The model under review builds one solid part; all positions refer to its coordinate system, in mm. A direction names the side the tool comes from. Give positions to 0.01 mm unless a question says otherwise; leave off trailing zeros. Loops run counter-clockwise (first coordinate to the right, second up) from the corner with the lowest first, then second, coordinate; pieces in that order, holes last. Notation, with made-up numbers: M 46,-34 L 75,-34 A21 cw 75,-10 Z; hole C 51,-30.75 d10. An arc over 180 degrees is marked long. Put each result on its own line as item: value. Start each with the question number.
from build123d import *

# Parameters (mm, degrees)
SKETCH1_W           = 10.541
SKETCH1_H           = 14.732
BOSS_EXTRUDE1_DEPTH = 1.524
SKETCH2_W           = 6.35
SKETCH2_H           = 9.652
BOSS_EXTRUDE2_DEPTH = 2.032
CUT_EXTRUDE1_DEPTH  = 6.35


with BuildPart() as part:
    # Sketch1 → Boss-Extrude1 (new body)
    with BuildSketch(Plane(origin=(0, 0, 0), x_dir=(0, 0, -1), z_dir=(1, 0, 0))):
        Rectangle(SKETCH1_W, SKETCH1_H)
    extrude(amount=BOSS_EXTRUDE1_DEPTH)

    # Sketch2 → Boss-Extrude2 (add)
    with BuildSketch(Plane(origin=(1.524, 0, 0), x_dir=(0, 0, -1), z_dir=(1, 0, 0))):
        Rectangle(SKETCH2_W, SKETCH2_H)
    extrude(amount=BOSS_EXTRUDE2_DEPTH)

    # Sketch3 → Cut-Extrude1 (cut)
    with BuildSketch(Plane.XY.offset(3.175)):
        Polygon((1.524, -4.826), (3.556, -3.234816243), (2.306647012, 0), (1.524, 4.826), (4.824013739, 4.826), (4.824013739, -4.826), align=None)
    extrude(amount=-CUT_EXTRUDE1_DEPTH, mode=Mode.SUBTRACT)


solid = part.part
(1) For faces 1 (the flat face through (2, -1, -3.175)), 2 (the flat face through (2, -1, 3.175)), 3 (the flat face through (0, 0, 0)), list the 3-axis set-ups (+Z, -Z, +X, -X, +Y, -Y) from which the entire face can be reached by the end or side of a thin tool; tool diameter is ignored.
(2) We need section D-D, the plane y = 6.75. Write out the cut boundary in (x, z).
(3) We need section B-B, the plane y = -2.5. Write out the cut boundary in (x, z) (1 decimal).
(4) We need section C-C, the plane x = 2.5. Write out the cut boundary in (y, z) (3 decimals).
(5) Insertion check: pin 1 (3 mm diameter, centred on y = 3.5, z = -1.5, fed in from +X); pin 2 (1.5 mm diameter, centred on x = 3, z = 0.5, fed in from -Y). Each pin has a flat end and moves straight along its axis. Give the tip position at first contact, or say it passes through.
(6) To check wall thickness, follow L1, parallel to X at y = -5.75, z = 2.25; L2, parallel to Z at x = 1.9, y = -4 (3 decimals); L3, parallel to X at y = -0.25, z = 0. State the ranges of each line that lie inside material, in increasing order. Write a range as [from, to].
(7) We need section A-A, the plane z = -1.5. Write out the cut boundary in (x, y), plus the area to 3 significant figures.
Check sheet entries:
1. face 1: -Z, +X, +Y, -Y
1. face 2: +Z, +X, +Y, -Y
1. face 3: +Z, -Z, -X, +Y, -Y
2. outline: M 0,-5.27 L 1.52,-5.27 L 1.52,5.27 L 0,5.27 Z
3. outline: M 0,-5.3 L 1.5,-5.3 L 1.5,-3.2 L 3.3,-3.2 L 3.3,3.2 L 1.5,3.2 L 1.5,5.3 L 0,5.3 Z
4. outline: M -4.062,-3.175 L -0.501,-3.175 L -0.501,3.175 L -4.062,3.175 Z
5. pin 1: stops at x = 1.98
5. pin 2: stops at y = -4.26
6. L1: x = [0, 1.52]
6. L2: z = [-3.175, 3.175]
6. L3: x = [0, 2.4]
7. outline: M 0,-7.37 L 1.52,-7.37 L 1.52,-4.83 L 3.56,-3.23 L 2.31,0 L 1.52,4.83 L 1.52,7.37 L 0,7.37 Z
7. area: 30.5 mm²
